Geometry: see drawing. Coordinates: mm, zero at the bounding-box minimum. A direction names the side the tool comes from. Give positions to 0.01 mm unless a question says otherwise; leave off trailing zeros. Write each loop counter-clockwise with the first axis right and the second up, starting at its lowest first coordinate (ties: lowest second). Pieces come first, ordered by that corner, then holes. Notation, with made-up numbers: (59, -13) - (84, -13) arc R21 cw to (84, 25) - close; hole circle Ø8 at (8.25, -11.5). An arc over 180 degrees is marked (long way). Use a Markdown table: item, result. Add a question column.
1. Section query A-A, the plane x = 22.5. Return loops of the section in (y, z).
2. Section query D-D, the plane z = 34.5. Return loops of the section in (x, y).
3. Material intervals for probe 1 along X at (y, z) = (1.8, 22.5) (1 decimal); probe 2 along X at (y, z) = (0.3, 23) (1 decimal); probe 3 along X at (y, z) = (2.25, 38), sorted ascending.
4. Pin query (flat end, axial travel): pin 1 (6.5 mm diameter, centred on x = 7, z = 22.5, fed in from -Y); pin 2 (4 mm diameter, centred on x = 5.5, z = 22.5, fed in from +Y); pin 3 (3 mm diameter, centred on x = 30, y = 4.5, fed in from -Z) (1 decimal); pin 4 (3 mm diameter, centred on y = 2, z = 23.5, fed in from -X). Return the tip coordinate at first contact, or that it passes through.
5. Mould query, pull axis X, two halves, no side actions, for the marked faces 3, 4 and 5. Classes: released by +X, released by -X, zero draft, split by the parting line, or undercut.
6. Section query C-C, the plane z = 39. Return loops of the section in (x, y).
7. Set-up query: the marked faces 1 and 2. Return all of +Z, -Z, +X, -X, +Y, -Y with unobstructed straight access to the full face (end or side cutting, diameter ignored); none if empty.
8. Section query B-B, the plane x = 27.5. Return loops of the section in (y, z).
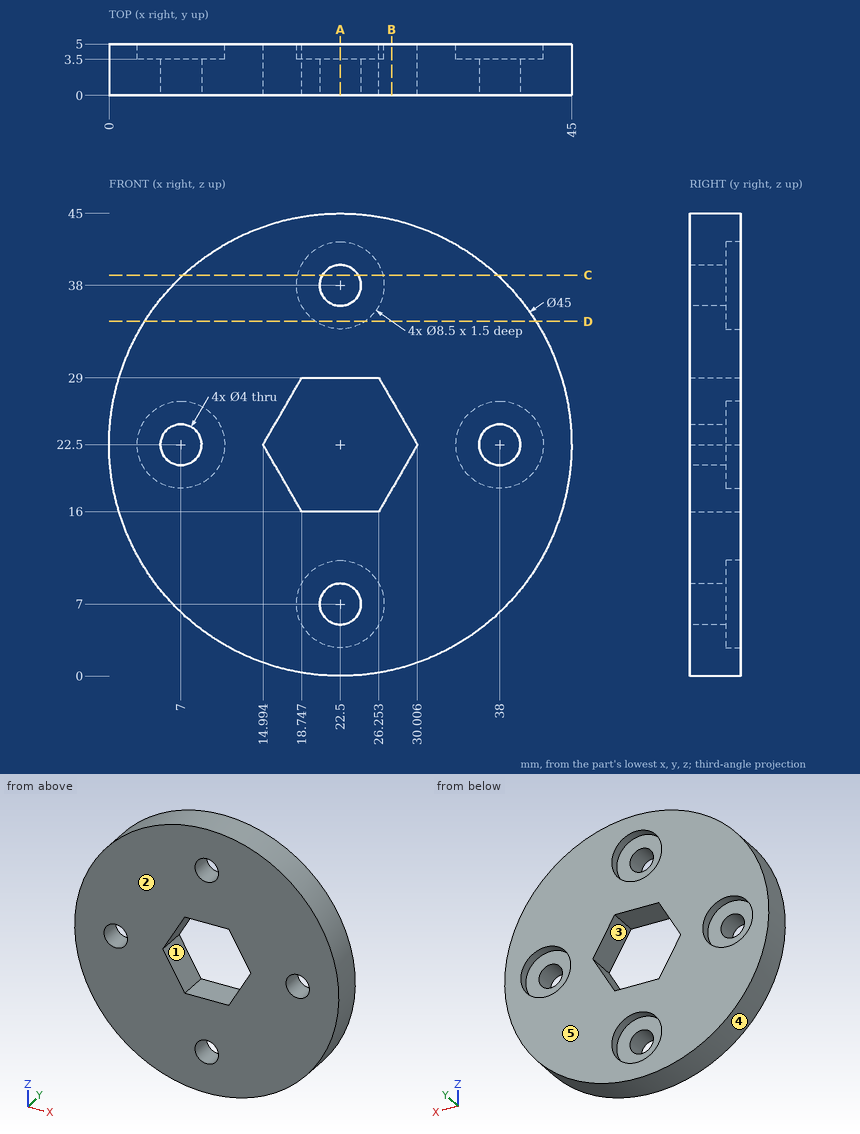
Result sheet:
| question | item | result |
|---|---|---|
| 1 | outline | (0, 0) - (5, 0) - (5, 2.75) - (3.5, 2.75) - (3.5, 5) - (0, 5) - close; (0, 9) - (3.5, 9) - (3.5, 11.25) - (5, 11.25) - (5, 16) - (0, 16) - close; (0, 29) - (5, 29) - (5, 33.75) - (3.5, 33.75) - (3.5, 36) - (0, 36) - close; (0, 40) - (3.5, 40) - (3.5, 42.25) - (5, 42.25) - (5, 45) - (0, 45) - close |
| 2 | outline | (3.47, 0) - (41.53, 0) - (41.53, 5) - (24.91, 5) - (24.91, 3.5) - (20.09, 3.5) - (20.09, 5) - (3.47, 5) - close |
| 3 | probe 1 | x = 0 to 5, 9 to 15, 30 to 36, 40 to 45 |
| 3 | probe 2 | x = 0 to 5.1, 8.9 to 15.3, 29.7 to 36.1, 39.9 to 45 |
| 3 | probe 3 | x = 6.19 to 20.5, 24.5 to 38.81 |
| 4 | pin 1 | stops at y = 0 |
| 4 | pin 2 | stops at y = 3.5 |
| 4 | pin 3 | stops at z = 0.8 |
| 4 | pin 4 | stops at x = 0 |
| 5 | face 3 | undercut |
| 5 | face 4 | split by the parting line |
| 5 | face 5 | zero draft |
| 6 | outline | (7.2, 0) - (20.77, 0) - (20.77, 3.5) - (18.37, 3.5) - (18.37, 5) - (7.2, 5) - close; (24.23, 0) - (37.8, 0) - (37.8, 5) - (26.63, 5) - (26.63, 3.5) - (24.23, 3.5) - close |
| 7 | face 1 | +Y, -Y |
| 7 | face 2 | +Z, -Z, +X, -X, -Y |
| 8 | outline | (0, 0.56) - (5, 0.56) - (5, 18.16) - (0, 18.16) - close; (0, 26.84) - (5, 26.84) - (5, 44.44) - (0, 44.44) - close |
